Autodesk Inventor part; units mm, degrees
ref_plane "YZ Plane" through (0, 0, 0) normal (1, 0, 0) x (0, 1, 0)
ref_plane "XZ Plane" through (0, 0, 0) normal (0, 1, 0) x (-1, 0, 0)
ref_plane "XY Plane" through (0, 0, 0) normal (0, 0, 1) x (1, 0, 0)
sketch "スケッチ1" plane through (0, 0, 0) normal (0, 0, 1) x (1, 0, 0)
  line L0 (-231, 344) -> (231, 344)
  line L1 (231, 344) -> (231, -344)
  line L2 (231, -344) -> (-231, -344)
  line L3 (-231, -344) -> (-231, 344)
  line L4 (-231, 344) -> (231, -344) construction
  line L5 (231, 344) -> (-231, -344) construction
  point P0 (0, 0)
  dimension "d0" = 462
  dimension "d1" = 688
extrude "押し出し1" add sketch "スケッチ1" along normal blind 8.35
sketch "スケッチ2" plane through (0, 0, 8.35) normal (0, 0, 1) x (1, 0, 0)
  line L0 (-200, -314.5) -> (200, -314.5)
  line L1 (200, -314.5) -> (200, 314.5)
  line L2 (200, 314.5) -> (-200, 314.5)
  line L3 (-200, 314.5) -> (-200, -314.5)
  line L4 (-200, -314.5) -> (200, 314.5) construction
  line L5 (200, -314.5) -> (-200, 314.5) construction
  point P0 (0, 0)
  dimension "d4" = 400
  dimension "d5" = 629
extrude "押し出し2" cut sketch "スケッチ2" against normal blind 8.35
fillet "フィレット1" radius 3 11 edges at (231, 344, 4.175) (231, 0, 8.35) (0, 344, 8.35) (0, 344, 0) (231, 0, 0) (-231, 344, 4.175) (-231, 0, 8.35) (-231, 0, 0) (-231, -344, 4.175) (0, -344, 8.35) (0, -344, 0)
properties part number "lowerGom"
The listing builds one solid part. Answer for the finished solid, in the listing's coordinates (mm). Give positions to 0.01 mm unless a question says otherwise; leave off trailing zeros. Write each loop counter-clockwise with the first axis right and the second up, starting at its lowest first coordinate (ties: lowest second). Pieces come first, ordered by that corner, then holes. Notation, with made-up numbers: (-13, 63) - (33, 63) arc R33 ccw to (33, 97) - close; hole circle Ø3 at (-8.75, 79.25). An arc over 180 degrees is marked (long way). One line per question, with ' | ' between items. Start each with the question number.
1. Section A-A, the plane x = -188 is taken. Determine the outline of the cut face in (y, z).
2. Section B-B, the plane y = -296 is taken. Determine the outline of the cut face in (x, z), then the cut area to 3 significant figures.
3. Straight lines are drawn through the part: line 1 (Y direction, x = 10, z = 4.5); line 2 (X direction, y = -229, z = 6); line 3 (X direction, y = 274, z = 5.5). For each, find the intervals that lie inside material, in ascending order.
4. Section C-C, the plane z = 7 is taken. Determine the outline of the cut face in (x, y), then the cut area to 3 significant figures.
Result:
1) outline: (-344, 3) arc R3 ccw to (-341, 0) - (-314.5, 0) - (-314.5, 8.35) - (-341, 8.35) arc R3 ccw to (-344, 5.35) - close; (314.5, 0) - (341, 0) arc R3 ccw to (344, 3) - (344, 5.35) arc R3 ccw to (341, 8.35) - (314.5, 8.35) - close
2) outline: (-231, 3) arc R3 ccw to (-228, 0) - (-200, 0) - (-200, 8.35) - (-228, 8.35) arc R3 ccw to (-231, 5.35) - close; (200, 0) - (228, 0) arc R3 ccw to (231, 3) - (231, 5.35) arc R3 ccw to (228, 8.35) - (200, 8.35) - close | area: 510 mm2
3) line 1: y = -344 to -314.5, 314.5 to 344 | line 2: x = -230.93 to -200, 200 to 230.93 | line 3: x = -231 to -200, 200 to 231
4) outline: (-230.51, -341) arc R2.51 ccw to (-228, -343.51) - (230.51, -343.51) - (230.51, 341) arc R2.51 ccw to (228, 343.51) - (-228, 343.51) arc R2.51 ccw to (-230.51, 341) - close; hole (-200, -314.5) - (200, -314.5) - (200, 314.5) - (-200, 314.5) - close | area: 65,100 mm2
